```python
from build123d import *

# Parameters (mm, degrees)
SKETCH_1_R      = 4
EXTRUDE_1_DEPTH = 5
CHAMFER_1_SIZE  = 0.5


with BuildPart() as part:
    # 草图1 → 凸台-拉伸1 (new body)
    with BuildSketch(Plane.XY):
        Polygon((0, 7.505553499), (-6.5, 3.75277675), (-6.5, -3.75277675), (0, -7.505553499), (6.5, -3.75277675), (6.5, 3.75277675), align=None)
        Circle(SKETCH_1_R, mode=Mode.SUBTRACT)
    extrude(amount=EXTRUDE_1_DEPTH)

    # 草图2 → 切除-旋转1 (revolve, cut)
    with BuildSketch(Plane(origin=(0, 0, 0), x_dir=(0, 0, -1), z_dir=(1, 0, 0)), mode=Mode.PRIVATE) as cut_revolve_1_sk:
        Polygon((-4.142378968, 7.640341523), (-5.294673063, 5.938491783), (-5.294673063, 7.640341523), align=None)
    cut_revolve_1 = revolve(cut_revolve_1_sk.sketch.rotate(Axis((0, 0, 5), (0, 0, -1)), 300.000000026), axis=Axis((0, 0, 5), (0, 0, -1)), mode=Mode.SUBTRACT)

    # 镜向2: 切除-旋转1 across plane
    add(cut_revolve_1.mirror(Plane(origin=(0, 0, 2.5), x_dir=(1, 0, 0), z_dir=(0, 0, -1))), mode=Mode.SUBTRACT)

    # 倒角1
    chamfer_1_edges = [part.edges().sort_by_distance(p)[0] for p in [
        (-4, 0, 0),
        (-4, 0, 5),
    ]]
    chamfer(chamfer_1_edges, length=CHAMFER_1_SIZE)


solid = part.part
```
Part model, mm, in its own coordinate system. Round coordinates to 2 decimals unless told otherwise and drop trailing zeros. Loops run counter-clockwise (first coordinate to the right, second up) from the corner with the lowest first, then second, coordinate; pieces in that order, holes last.
1. Flat gauge pin, fed straight in: pin 1 (3 mm diameter, centred on y = 5.5, z = 4, fed in from +X). Where does the tip first touch, or does it go through?
Solutions:
pin 1: stops at x = 6.07
2. Drill centre lines: line 1 along X through (y, z) = (-3.5, 4.75); line 2 along X through (y, z) = (-2.5, 1.9); line 3 along Y through (x, z) = (-2.25, 1.6). Where is each one in solid material? Low to high.
Solutions:
line 1: x = -5.76 to -2.41, 2.41 to 5.76
line 2: x = -6.5 to -3.12, 3.12 to 6.5
line 3: y = -6.21 to -3.31, 3.31 to 6.21
3. Two-plate mould, pull along Y, no slides. Class faces 1 (the face through (-0.867, -3.905, 2.472)), 2 (the face through (-6.5, 0, 2)), 3 (the face through (3.2, -5.66, 2.47)): pulls with the +Y half, pulls with the -Y half, needs draft (parallel to the pull), parting line crosses it, or undercut.
Solutions:
face 1: undercut
face 2: needs draft
face 3: pulls with the -Y half
4. Slice it at A-A (z = 1.7). Give the cut face in (x, y).
Solutions:
outline: (-6.5, -3.75) - (0, -7.51) - (6.5, -3.75) - (6.5, 3.75) - (0, 7.51) - (-6.5, 3.75) - close; hole circle Ø8 at (0, 0)
5. Slice it at B-B (y = 0). Give the cut face in (x, z).
Solutions:
outline: (-6.5, 0.09) - (-6.37, 0) - (-4.5, 0) - (-4, 0.5) - (-4, 4.5) - (-4.5, 5) - (-6.37, 5) - (-6.5, 4.91) - close; (4, 0.5) - (4.5, 0) - (6.37, 0) - (6.5, 0.09) - (6.5, 4.91) - (6.37, 5) - (4.5, 5) - (4, 4.5) - close
